Can you work these out from the model? Positions are in its coordinate system, mm. A direction names the side the tool comes from. Round coordinates to 2 decimals unless told otherwise and drop trailing zeros. Write each loop counter-clockwise with the first axis right and the second up, starting at its lowest first coordinate (ties: lowest second). Pieces come first, ordered by that corner, then holes.
Q1. We'd pull the mould along X, two halves only. Please class faces 5 (the flat face through (10, -37, -103)), 6 (the cylindrical face through (23.977, 1.055, -283.986)), 7 (the flat face through (0, 29.686, -171)): +X half, -X half, draft (parallel to the pull), parting line (faces both ways), or undercut.
Q2. For faces 1 (the flat face through (26.1, 9.3, -100)), 2 (the flat face through (-5, 35, -171)), 3 (the cylindrical face through (-1.601, -37.966, -103.986)), 4 (the cylindrical face through (23.846, -7.509, -287.465)), which set-ups out of +Z, -Z, +X, -X, +Y, -Y let a thin tool reach every point of the face, with its end or its side?
Q3. Please list where these lines run through material, in increasing order: line 1 along Z through (x, y) = (-24.5, 4); line 2 along Z through (x, y) = (-29, -7.5); line 3 along Y through (x, z) = (1.5, -240.5).
Q4. If we section it at B-B (x = 32): Please give me the cut outline in (y, z), plus the area to 3 significant figures.
Q5. If we section it at C-C (z = -242): Please give me the cut outline in (x, y).
Q6. If we section it at A-A (z = -64): Please give me the cut outline in (x, y).
Q7. I'm going to push flat-ended pins straight in: pin 1 Ø11 at (y, z) = (32, -148.5) entering from -X; pin 2 Ø2 at (y, z) = (-3, -180) entering from +X; pin 3 Ø4 at (y, z) = (-23.5, -173) entering from +X. Where does each tip first touch, or does it pass through?
from build123d import *

# Parameters (mm, degrees)
ESQUISSE1_R             = 25
BOSS_EXTRU_1_DEPTH      = 100
BOSS_EXTRU_3_DEPTH      = 150
ESQUISSE5_R             = 25
BOSS_EXTRU_4_DEPTH      = 40
ESQUISSE6_R             = 27.5
BOSS_EXTRU_5_DEPTH      = 2
CONG_2_R                = 2.1
CONG_3_R                = 2.1
ESQUISSE7_R             = 25
ESQUISSE7_R_2           = 24
ENL_V_MAT_EXTRU_1_DEPTH = 2
BOSS_EXTRU_6_START      = -5
BOSS_EXTRU_6_DEPTH      = 5
ENL_V_START             = 2
ESQUISSE10_R            = 40
ESQUISSE10_R_2          = 38
ENL_V_MAT_EXTRU_2_DEPTH = 2


with BuildPart() as part:
    # Esquisse1 → Boss.-Extru.1 (new body)
    with BuildSketch(Plane.XY):
        Circle(ESQUISSE1_R)
    extrude(amount=-BOSS_EXTRU_1_DEPTH)

    # Esquisse4 → Boss.-Extru.3 (add)
    with BuildSketch(Plane(origin=(0, 0, -100), x_dir=(-1, 0, 0), z_dir=(0, 0, -1))):
        with BuildLine():
            Line((-5, 39.686269666), (-5, 29.686269666))
            Line((-5, 29.686269666), (5, 29.686269666))
            Line((5, 29.686269666), (5, 39.686269666))
            ThreePointArc((5, 39.686269666), (0, -40), (-5, 39.686269666))
        make_face()
    extrude(amount=BOSS_EXTRU_3_DEPTH)

    # Esquisse5 → Boss.-Extru.4 (add)
    with BuildSketch(Plane(origin=(0, 0, -250), x_dir=(-1, 0, 0), z_dir=(0, 0, -1))):
        with Locations(Location((0, 0, 0), (0, 0, 180))):
            Circle(ESQUISSE5_R)
    extrude(amount=BOSS_EXTRU_4_DEPTH)

    # Esquisse6 → Boss.-Extru.5 (add)
    with BuildSketch(Plane.XY.offset(-100)):
        with Locations(Location((0, 0, 0), (0, 0, 180))):
            Circle(ESQUISSE6_R)
    boss_extru_5 = extrude(amount=BOSS_EXTRU_5_DEPTH)

    # Congé2
    cong_2_edges = [part.edges().sort_by_distance(p)[0] for p in [
        (-25, 0, -98),
    ]]
    fillet(cong_2_edges, radius=CONG_2_R)

    # Symétrie3: Boss.-Extru.5 across plane
    add(boss_extru_5.mirror(Plane.XY.offset(-175)))

    # Congé3
    cong_3_edges = [part.edges().sort_by_distance(p)[0] for p in [
        (-25, 0, -252),
    ]]
    fillet(cong_3_edges, radius=CONG_3_R)

    # Esquisse7 → Enlèv. mat.-Extru.1 (cut)
    with BuildSketch(Plane(origin=(0, 0, -283), x_dir=(-1, 0, 0), z_dir=(0, 0, -1))):
        Circle(ESQUISSE7_R)
        Circle(ESQUISSE7_R_2, mode=Mode.SUBTRACT)
    extrude(amount=ENL_V_MAT_EXTRU_1_DEPTH, mode=Mode.SUBTRACT)

    # Esquisse9 → Boss.-Extru.6 (add)
    with BuildSketch(Plane(origin=(0, 0, -250), x_dir=(-1, 0, 0), z_dir=(0, 0, -1)).offset(BOSS_EXTRU_6_START)):
        with BuildLine():
            ThreePointArc((-5, 39.686269666), (0, 40), (5, 39.686269666))
            Line((5, 39.686269666), (5, 29.686269666))
            Line((5, 29.686269666), (-5, 29.686269666))
            Line((-5, 29.686269666), (-5, 39.686269666))
        make_face()
    extrude(amount=BOSS_EXTRU_6_DEPTH)

    # Esquisse10 → Enlèv. mat.-Extru.2 (cut)
    with BuildSketch(Plane.XY.offset(-105).offset(ENL_V_START)):
        with Locations(Location((0, 0, 0), (0, 0, 82.819244219))):
            Circle(ESQUISSE10_R)
        Circle(ESQUISSE10_R_2, mode=Mode.SUBTRACT)
    extrude(amount=-ENL_V_MAT_EXTRU_2_DEPTH, mode=Mode.SUBTRACT)


solid = part.part
A:
1. face 5: draft
1. face 6: parting line
1. face 7: undercut
2. face 1: +Z
2. face 2: +Z, +Y
2. face 3: none
2. face 4: -Z
3. line 1: z = -290 to -285, -283 to 0
3. line 2: z = -250 to -100
3. line 3: y = -39.97 to 29.69
4. outline: (-24, -250) - (24, -250) - (24, -105) - (20.49, -105) - (20.49, -103) - (24, -103) - (24, -100) - (-24, -100) - (-24, -103) - (-20.49, -103) - (-20.49, -105) - (-24, -105) - close
4. area: 7,190 mm2
5. outline: (-5, 29.69) - (-5, 39.69) arc R40 ccw (long way) to (5, 39.69) - (5, 29.69) - close
6. outline: circle Ø50 at (0, 0)
7. pin 1: stops at x = -29.96
7. pin 2: stops at x = 39.95
7. pin 3: stops at x = 33.73
